Check sheet for the drawn part. Datum: minimum x, y, z corner. Units: mm. A direction names the side the tool comes from. Give positions to 0.01 mm unless a question says otherwise; leave off trailing zeros. Loops run counter-clockwise (first coordinate to the right, second up) from the corner with the lowest first, then second, coordinate; pieces in that order, holes last. Notation, with made-up numbers: (11.25, 12) - (56.25, 12) arc R14 ccw to (56.25, 18) - close; hole circle Ø3 at (89.25, 45). An arc over 180 degrees is marked (long way). Use one line per item in the form item = value.
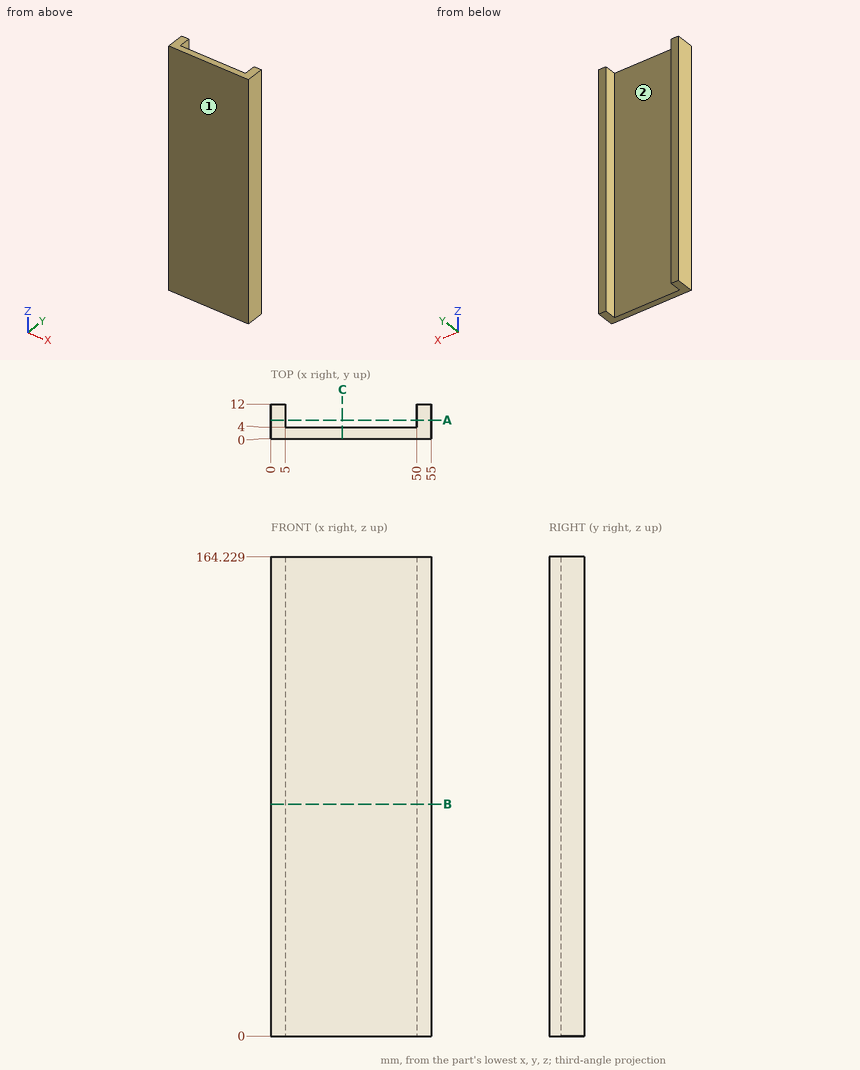
Item 1: Section check B-B on z = 79.5. Record the boundary of the cut face in (x, y).
Answer block:
outline = (0, 0) - (55, 0) - (55, 12) - (50, 12) - (50, 4) - (5, 4) - (5, 12) - (0, 12) - close
Item 2: Gauge pin test, flat ends, axial feed: P1, Ø4, axis at y = 9, z = 106.5, coming from the -X side; P2, Ø1, axis at x = 7.5, z = 97, coming from the +Y side. Record the tip position at first contact, or that the pin passes through.
Answer block:
P1 = 0
P2 = 4
Item 3: Section check A-A on y = 6.5. Record the boundary of the cut face in (x, z), then the cut area to 3 significant figures.
Answer block:
outline = (0, 0) - (5, 0) - (5, 164.23) - (0, 164.23) - close; (50, 0) - (55, 0) - (55, 164.23) - (50, 164.23) - close
area = 1,640 mm2
Item 4: Section check C-C on x = 24.5. Record the boundary of the cut face in (y, z), then the cut area to 3 significant figures.
Answer block:
outline = (0, 0) - (4, 0) - (4, 164.23) - (0, 164.23) - close
area = 657 mm2
Item 5: Thickness scan on L1, parallel to X at y = 10, z = 95; L2, parallel to Y at x = 35.5, z = 60.5. Record the ranges inside material, lowest first.
Answer block:
L1 = 0 to 5, 50 to 55
L2 = 0 to 4
Item 6: Access from +Z, -Z, +X, -X, +Y, -Y to the whole of each face (thin tool, end or side, straight path). Record for the marked faces 1 and 2.
Answer block:
face_1 = +Z, -Z, +X, -X, -Y
face_2 = +Z, -Z, +Y
